Geometry check sheet. Reference: the model listing, model coordinates, mm. A direction names the side the tool comes from. Round coordinates to 2 decimals unless told otherwise and drop trailing zeros. Order: outer loops, then holes, each group sorted by start corner. A loop starts at its lowest first (then second) coordinate and runs counter-clockwise, first axis right, second up. Notation, with made-up numbers: (-21.5, 25.5) - (-15.5, 25.5) arc R4 cw to (-15.5, 29.5) - close; hole circle Ø11 at (80, -38.75). An arc over 180 degrees is marked (long way). Return JSON: item names as keys, results as strings. Group by question number.
Q1. Sectioned sample at C-C, the plane x = -38.5. Record the cut outline in (y, z), then the cut area to 3 significant figures.
Q2. Sectioned sample at A-A, the plane y = 3. Record the cut outline in (x, z).
Q3. Sectioned sample at B-B, the plane z = -71. Record the cut outline in (x, y).
Q4. Material ranges on line 1 along X through (y, z) = (8.25, -73); line 2 along Z through (x, y) = (-35, 3.75); line 3 along Z through (x, y) = (-44, 1.25), recorded low to high.
Q5. Gauge pin test, flat ends, axial feed: pin 1 Ø4 at (y, z) = (6.5, -5) entering from +X; pin 2 Ø1.9 at (x, z) = (-53.14, -84.37) entering from +Y; pin 3 Ø5 at (x, y) = (-36, 2) entering from -Z. Record the tip position at first contact, or that the pin passes through.
Q6. Draft check along X on faces 1 (the flat face through (-48.14, 5, -50)), 2 (the flat face through (-53, 5, -104.367)), 3 (the cylindrical face through (-54.622, 5.07, -44.714)). Enter one of: pulls with the +X half, pulls with the -X half, needs draft (parallel to the pull), parting line crosses it, or undercut.
Q7. Tool access check on faces 4 (the flat face through (-40, 5, 17.786)), 5 (the flat face through (-40, 5, 6.786)). Record the directions out of +Z, -Z, +X, -X, +Y, -Y that give a thin tool (end or side, any length) a straight path to the whole face; none if there is none.
```python
from build123d import *

# Parameters (mm, degrees)
BOSS_EXTRUDE1_DEPTH  = 10
FILLET1_R            = 10
M3_CLEARANCE_HOLE1_D = 3.2


with BuildPart() as part:
    # Sketch1 → Boss-Extrude1 (new body)
    with BuildSketch(Plane(origin=(0, 0, 0), x_dir=(1, 0, 0), z_dir=(0, 1, 0))):
        with BuildLine():
            Line((-58.140357718, 104.367316493), (-48.140357718, 104.367316493))
            Line((-48.140357718, 104.367316493), (-48.140357718, -6.785904903))
            Line((-48.140357718, -6.785904903), (-32.275583784, -6.785904903))
            ThreePointArc((-32.275583784, -6.785904903), (-26.775583784, -12.285904903), (-32.275583784, -17.785904903))
            Line((-32.275583784, -17.785904903), (-58.140357718, -17.785904903))
            Line((-58.140357718, -17.785904903), (-58.140357718, -6.785904903))
            Line((-58.140357718, -6.785904903), (-58.140357718, 104.367316493))
        make_face()
    extrude(amount=BOSS_EXTRUDE1_DEPTH)

    # Fillet1
    fillet1_edges = [part.edges().sort_by_distance(p)[0] for p in [
        (-58.140357718, 5, 17.785904903),
    ]]
    fillet(fillet1_edges, radius=FILLET1_R)

    # M3 Clearance Hole1 (through all)
    with Locations(Plane(origin=(-35.775583784, 0, 12.285904903), x_dir=(0, 0, -1), z_dir=(0, -1, 0))):
        with Locations((0, 0), (96.653221396, -17.364773934), (56.653302681, -17.284133769)):
            Hole(M3_CLEARANCE_HOLE1_D / 2)


solid = part.part
```
Reply:
{
 "1": {"outline": "(0, 6.79) - (10, 6.79) - (10, 17.79) - (0, 17.79) - close", "area": "110 mm^2"},
 "2": {"outline": "(-58.14, -104.37) - (-48.14, -104.37) - (-48.14, 6.79) - (-32.28, 6.79) arc R5.5 ccw to (-32.28, 17.79) - (-48.14, 17.79) arc R10 ccw to (-58.14, 7.79) - close; hole circle Ø3.2 at (-53.14, -84.37); hole circle Ø3.2 at (-53.06, -44.37); hole circle Ø3.2 at (-35.78, 12.29)"},
 "3": {"outline": "(-58.14, 0) - (-48.14, 0) - (-48.14, 10) - (-58.14, 10) - close"},
 "4": {"line 1": "-58.14 to -48.14", "line 2": "6.79 to 10.89, 13.69 to 17.79", "line 3": "6.79 to 17.79"},
 "5": {"pin 1": "x = -48.14", "pin 2": "through", "pin 3": "z = 6.79"},
 "6": {"face 1": "pulls with the +X half", "face 2": "needs draft", "face 3": "undercut"},
 "7": {"face 4": "+Z, +X, -X, +Y, -Y", "face 5": "-Z, +X, +Y, -Y"}
}
